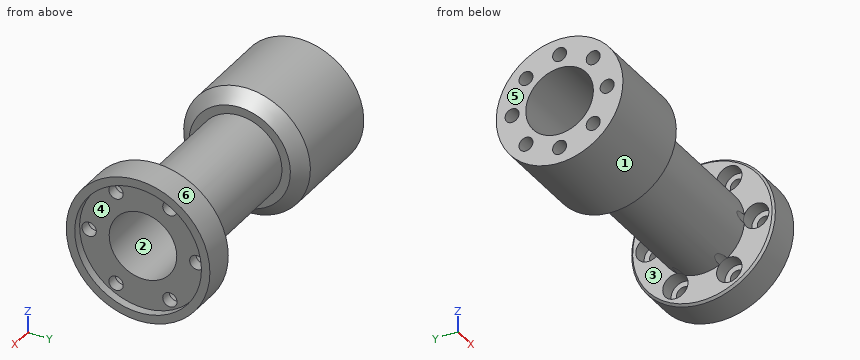
from build123d import *

# Parameters (mm, degrees)
SKETCH_2_R               = 8
CUT_EXTRUDE_1_DEPTH      = 71.524392943
SKETCH_6_R               = 3
PATTERN_CIRCULAR_2_COUNT = 6
SKETCH_5_R               = 15
CUT_EXTRUDE_2_DEPTH      = 2
CHAMFER_1_SIZE           = 3
CHAMFER_2_SIZE           = 0.5
PATTERN_CIRCULAR_3_COUNT = 8


with BuildPart() as part:
    # Sketch 1 → Revolve 1 (revolve)
    with BuildSketch(Plane(origin=(0, 0, 0), x_dir=(1, 0, 0), z_dir=(0, 1, 0)), mode=Mode.PRIVATE) as revolve_1_sk:
        Polygon((0, 0), (0, 15), (24.8, 15), (24.8, 10), (58.3, 10), (58.3, 17), (66.3, 17), (66.3, 0), align=None)
    revolve(revolve_1_sk.sketch.rotate(Axis((-27.673469388, 0, 0), (1, 0, 0)), 180), axis=Axis((-27.673469388, 0, 0), (1, 0, 0)))

    # Sketch 2 → Cut-Extrude 1 (cut, through all)
    with BuildSketch(Plane.ZY):
        Circle(SKETCH_2_R)
    extrude(amount=-CUT_EXTRUDE_1_DEPTH, mode=Mode.SUBTRACT)

    # Sketch 3 → Hole Wizard 1 (revolve, cut)
    with BuildSketch(Plane(origin=(58.3, 12.75, 0), x_dir=(0, 0, 1), z_dir=(0, 1, 0))):
        Polygon((0, 0), (0, 8), (1.7, 8), (1.7, 3.4), (3, 3.4), (3, 0), align=None)
    hole_wizard_1 = revolve(axis=Axis((51.95, 12.75, 0), (1, 0, 0)), mode=Mode.SUBTRACT)

    # Sweep 1: sweep along a path in Sketch 7
    with BuildLine(Plane.XY) as sweep_1_path:
        ThreePointArc((58.3, 13.946689979), (47.696988858, 17.813586648), (42.072772548, 27.598520272))
    # Sketch 6 → Sweep 1 (sweep, cut)
    with BuildSketch(Plane.ZY.offset(-58.3)):
        with Locations((0, 12.75)):
            Circle(SKETCH_6_R)
    sweep_1 = sweep(path=sweep_1_path.line, mode=Mode.SUBTRACT)

    # Pattern Circular 2: Hole Wizard 1, Sweep 1 ×6 about axis
    pattern_circular_2_axis = Axis((0, 0, 0), (1, 0, 0))
    add([hole_wizard_1.rotate(pattern_circular_2_axis, i * 360 / PATTERN_CIRCULAR_2_COUNT) for i in range(1, PATTERN_CIRCULAR_2_COUNT)], mode=Mode.SUBTRACT)
    add([sweep_1.rotate(pattern_circular_2_axis, i * 360 / PATTERN_CIRCULAR_2_COUNT) for i in range(1, PATTERN_CIRCULAR_2_COUNT)], mode=Mode.SUBTRACT)

    # Sketch 5 → Cut-Extrude 2 (cut)
    with BuildSketch(Plane(origin=(66.3, 0, 0), x_dir=(0, 0, -1), z_dir=(1, 0, 0))):
        with Locations(Location((0, 0, 0), (0, 0, 180))):
            Circle(SKETCH_5_R)
    extrude(amount=-CUT_EXTRUDE_2_DEPTH, mode=Mode.SUBTRACT)

    # Chamfer 1
    chamfer_1_edges = [part.edges().sort_by_distance(p)[0] for p in [
        (24.8, 0, -15),
    ]]
    chamfer(chamfer_1_edges, length=CHAMFER_1_SIZE)

    # Chamfer 2
    chamfer_2_edges = [part.edges().sort_by_distance(p)[0] for p in [
        (58.3, 0, -17),
    ]]
    chamfer(chamfer_2_edges, length=CHAMFER_2_SIZE)

    # Sketch 11 → Hole Wizard M4 _1 (revolve, cut)
    with BuildSketch(Plane.ZX.offset(11.25)):
        Polygon((0, 0), (0, 8.091420021), (1.65, 7.1), (1.65, 0), align=None)
    hole_wizard_m4_1 = revolve(axis=Axis((-6.35, 11.25, 0), (1, 0, 0)), mode=Mode.SUBTRACT)

    # Pattern Circular 3: Hole Wizard M4 _1 ×8 about axis
    pattern_circular_3_axis = Axis((0, 0, 0), (1, 0, 0))
    for i in range(1, PATTERN_CIRCULAR_3_COUNT):
        add(hole_wizard_m4_1.rotate(pattern_circular_3_axis, i * 360 / PATTERN_CIRCULAR_3_COUNT), mode=Mode.SUBTRACT)


solid = part.part
Verification items for the finished model (mm, model axes). Face numbers are marked on the shaded views. A direction names the side the tool comes from. Give positions to 0.01 mm unless a question says otherwise; leave off trailing zeros. Loops run counter-clockwise (first coordinate to the right, second up) from the corner with the lowest first, then second, coordinate; pieces in that order, holes last.
1) Depth check by flat-ended pin: pin 1 Ø4 at (x, z) = (36.5, 0) entering from +Y; pin 2 Ø1.5 at (y, z) = (2, -10) entering from +X; pin 3 Ø8 at (x, y) = (15, -5) entering from +Z. Enter the tip coordinate at first touch or a pass-through.
2) Thickness scan on line 1 along Y through (x, z) = (5.75, 0); line 2 along Y through (x, z) = (65, 0); line 3 along X through (y, z) = (-9, 1). Record the ranges inside material, lowest first.
3) Sectioned sample at A-A, the plane x = 39.5. Enter the section's corners in (y, z), then the cut area to 3 significant figures.
4) Set-up check for the marked faces 1, 2 and 3: record each of +Z, -Z, +X, -X, +Y, -Y from which the full face is reachable in a straight line by a thin tool's end or side.
5) Draft check along Z on the marked faces 4, 5 and 6. Enter one of: pulls with the +Z half, pulls with the -Z half, needs draft (parallel to the pull), parting line crosses it, or undercut.
6) Sectioned sample at B-B, the plane x = 61. Enter the section's corners in (y, z) (3 decimals).
Answers:
1. pin 1: stops at y = 10
1. pin 2: stops at x = 64.3
1. pin 3: stops at z = 14.97
2. line 1: y = -15 to -12.9, -9.6 to -8, 8 to 9.6, 12.9 to 15
2. line 2: y = -17 to -15, 15 to 17
2. line 3: x = 0 to 64.3
3. outline: circle Ø20 at (0, 0); hole circle Ø16 at (0, 0)
3. area: 113 mm2
4. face 1: -X
4. face 2: +X, -X
4. face 3: none
5. face 4: undercut
5. face 5: needs draft
5. face 6: parting line crosses it
6. outline: circle Ø34 at (0, 0); hole circle Ø6 at (-12.75, 0); hole circle Ø6 at (-6.375, -11.042); hole circle Ø6 at (-6.375, 11.042); hole circle Ø16 at (0, 0); hole circle Ø6 at (6.375, -11.042); hole circle Ø6 at (6.375, 11.042); hole circle Ø6 at (12.75, 0)
